Can you work these out from the model? Positions are in its coordinate system, mm. A direction names the side the tool comes from. Give positions to 0.01 mm unless a question says otherwise; leave off trailing zeros. Order: outer loops, then holes, each group sorted by start corner. A loop starts at its lowest first (then second) coordinate and runs counter-clockwise, first axis right, second up.
Item 1: I want a section at D-D, the plane y = -1. Write out the boundary of the cut face in (x, z), then the cut area to 3 significant figures.
Item 2: If we mould it in two halves opening along Y, with no side actions, what happens to faces 5 (the flat face through (-37, 0, 32.5)), 6 (the flat face through (-37, 10, 64.2)), 7 (the flat face through (-37, -15.45, 54)), 8 (the cylindrical face through (-37.48, 10.45, 37.38))? For each: +Y half, -Y half, draft (parallel to the pull), parting line (faces both ways), or undercut.
Item 3: Which directions (+Z, -Z, +X, -X, +Y, -Y) give clear straight access to the entire face, cutting with the end or side of a thin tool? Please do faces 1 (the flat face through (-35, 5, 45)), 2 (the flat face through (-32, 7.5, 66)), 3 (the flat face through (-57.5, 0, 51)), 4 (the flat face through (-56, 0, 52.1)).
Item 4: I want a section at A-A, the plane z = 54.5. Write out the boundary of the cut face in (x, y).
Item 5: I want a section at B-B, the plane x = -21. Write out the boundary of the cut face in (y, z).
Item 6: I'm going to push flat-ended pins straight in: pin 1 Ø4 at (y, z) = (-1, 40) entering from +X; pin 2 Ø2 at (y, z) = (0.5, 48.5) entering from +X; pin 3 Ø1.5 at (x, y) = (-44.5, -0.5) entering from +Z. Where does each tip first touch, or does it pass through?
Item 7: If I drill on line 1 along Y through (x, z) = (-48, 50.5); line 2 along Z through (x, y) = (-35, -0.5); line 3 along Z through (x, y) = (-50.5, -9.5), over which ranges is the centre line in solid material (lowest first)?
Item 8: I want a section at C-C, the plane z = 45.5. Write out the boundary of the cut face in (x, y).
```python
from build123d import *

# Parameters (mm, degrees)
SKETCH1_W               = 115
SKETCH1_H               = 90
BOSS_EXTRUDE1_DEPTH     = 2.5
SKETCH2_W               = 27.2
SKETCH2_H               = 30.9
SKETCH2_W_2             = 19.2
SKETCH2_H_2             = 22.9
BOSS_EXTRUDE2_DEPTH     = 40.6
SKETCH3_W               = 19.2
SKETCH3_H               = 22.9
BOSS_EXTRUDE3_DEPTH     = 4
CUT_EXTRUDE1_REACH      = 136.592
SKETCH4_W               = 5
SKETCH4_H               = 8
FILLET1_R               = 25
SKETCH5_W               = 38.2
SKETCH5_H               = 8
CUT_EXTRUDE2_DEPTH      = 39.6
CUT_EXTRUDE3_REACH      = 92.993
SKETCH6_W               = 20
SKETCH6_H               = 9.5
CUT_EXTRUDE4_REACH      = 129.903
CUT_EXTRUDE5_DEPTH      = 135.591762378
CUT_EXTRUDE5_DEPTH_BACK = 135.591762378
SKETCH9_W               = 100.7
SKETCH9_H               = 30.9
CUT_EXTRUDE6_REACH      = 92.993


# Read off the part's stored shape, not the designer's step: Mirror1
with BuildPart() as part:
    # Sketch1 → Boss-Extrude1 (new, symmetric)
    with BuildSketch(Plane(origin=(0, 0, 0), x_dir=(1, 0, 0), z_dir=(0, 1, 0))):
        Rectangle(SKETCH1_W, SKETCH1_H)
    extrude(amount=BOSS_EXTRUDE1_DEPTH, both=True)

    # Sketch2 → Boss-Extrude2 (add)
    with BuildSketch(Plane.ZY.offset(57.5)):
        with Locations((54.6, 0)):
            Rectangle(SKETCH2_W, SKETCH2_H)
        with Locations((54.6, 0)):
            Rectangle(SKETCH2_W_2, SKETCH2_H_2, mode=Mode.SUBTRACT)
    extrude(amount=-BOSS_EXTRUDE2_DEPTH)

    # Sketch3 → Boss-Extrude3 (add)
    with BuildSketch(Plane.ZY.offset(57.5)):
        with Locations((54.6, 0)):
            Rectangle(SKETCH3_W, SKETCH3_H)
    extrude(amount=-BOSS_EXTRUDE3_DEPTH)

    # Sketch4 → Cut-Extrude1 (cut, up to next)
    with BuildSketch(Plane.ZY.offset(57.5), mode=Mode.PRIVATE) as cut_extrude1_sk1:
        with Locations((54.6, 0)):
            Rectangle(SKETCH4_W, SKETCH4_H)
    cut_extrude1_tool1 = extrude(cut_extrude1_sk1.sketch, amount=-CUT_EXTRUDE1_REACH, mode=Mode.PRIVATE) & part.part
    add(cut_extrude1_tool1.solids().sort_by_distance((-57.5, 0, 54.6))[0], mode=Mode.SUBTRACT)

    # Fillet1
    # the kernel refuses this fillet: 25 mm, written as the material it adds along each edge
    with BuildSketch(Plane(origin=(-57.5, -2.5, 41), x_dir=(0, 0, -1), z_dir=(1, 0, 0))) as fillet1_piece_1:
        with BuildLine():
            CenterArc((21.904280404, -25), FILLET1_R, 90, 61.183893167)
            Line((0, -12.95), (-0.438085608, -12.709))
            ThreePointArc((-0.438085608, -12.709), (-0.5, -6.475), (-0.5, 0))
            Line((-0.5, 0), (0, 0.5))
            Line((0, 0.5), (21.904280404, 0.5))
            Line((21.904280404, 0.5), (21.904280404, 0))
        make_face()
    extrude(amount=40.6)
    with BuildSketch(Plane(origin=(-57.5, 2.5, 41), x_dir=(0, 0, -1), z_dir=(1, 0, 0))) as fillet1_piece_2:
        with BuildLine():
            CenterArc((21.904280404, 25), FILLET1_R, 208.816106833, 61.183893167)
            Line((0, 12.95), (-0.438085608, 12.709))
            ThreePointArc((-0.438085608, 12.709), (-0.5, 6.475), (-0.5, 0))
            Line((-0.5, 0), (0, -0.5))
            Line((0, -0.5), (21.904280404, -0.5))
            Line((21.904280404, -0.5), (21.904280404, 0))
        make_face()
    extrude(amount=40.6)

    # Sketch5 → Cut-Extrude2 (cut)
    with BuildSketch(Plane(origin=(-8.9, 0, 0), x_dir=(0, 0, -1), z_dir=(1, 0, 0))):
        with Locations((-54.6, 0)):
            Rectangle(SKETCH5_W, SKETCH5_H)
    extrude(amount=-CUT_EXTRUDE2_DEPTH, mode=Mode.SUBTRACT)

    # Sketch6 → Cut-Extrude3 (cut, up to next)
    with BuildSketch(Plane(origin=(0, 2.5, 0), x_dir=(1, 0, 0), z_dir=(0, 1, 0)), mode=Mode.PRIVATE) as cut_extrude3_sk1:
        with Locations((1.1, -40.25)):
            Rectangle(SKETCH6_W, SKETCH6_H)
    cut_extrude3_tool1 = extrude(cut_extrude3_sk1.sketch, amount=-CUT_EXTRUDE3_REACH, mode=Mode.PRIVATE) & part.part
    add(cut_extrude3_tool1.solids().sort_by_distance((1.1, 2.5, 40.25))[0], mode=Mode.SUBTRACT)

    # Sketch8 → Cut-Extrude4 (cut, up to next)
    with BuildSketch(Plane.XY.offset(68.2), mode=Mode.PRIVATE) as cut_extrude4_sk1:
        with BuildLine():
            Line((-46, 7.5), (-16, 7.5))
            ThreePointArc((-16, 7.5), (-8.5, 0), (-16, -7.5))
            Line((-16, -7.5), (-46, -7.5))
            ThreePointArc((-46, -7.5), (-53.5, 0), (-46, 7.5))
        make_face()
    cut_extrude4_tool1 = extrude(cut_extrude4_sk1.sketch, amount=-CUT_EXTRUDE4_REACH, mode=Mode.PRIVATE) & part.part
    add(cut_extrude4_tool1.solids().sort_by_distance((-31, 0, 68.2))[0], mode=Mode.SUBTRACT)

    # Mirror1
    split(bisect_by=Plane.XY, keep=Keep.TOP)

    # Mirror1 2: part across plane


with BuildPart() as part_1:
    add(part.part)
    add(part.part.mirror(Plane.XY))

    # Sketch9 → Cut-Extrude5 (cut, two sides: drawn at the far end of the back side and taken through both)
    with BuildSketch(Plane(origin=(57.5, 0, 0), x_dir=(0, 0, -1), z_dir=(1, 0, 0)).offset(-CUT_EXTRUDE5_DEPTH_BACK)):
        with Locations((17.85, 0)):
            Rectangle(SKETCH9_W, SKETCH9_H)
    extrude(amount=CUT_EXTRUDE5_DEPTH + CUT_EXTRUDE5_DEPTH_BACK, mode=Mode.SUBTRACT)

    # Sketch10 → Cut-Extrude6 (cut, up to next)
    with BuildSketch(Plane(origin=(0, 2.5, 0), x_dir=(1, 0, 0), z_dir=(0, 1, 0)), mode=Mode.PRIVATE) as cut_extrude6_sk1:
        Polygon((57.5, -32.5), (-16.9, -32.5), (-16.9, -35.5), (11.1, -35.5), (11.1, -45), (57.5, -45), align=None)
    cut_extrude6_tool1 = extrude(cut_extrude6_sk1.sketch, amount=-CUT_EXTRUDE6_REACH, mode=Mode.PRIVATE) & part_1.part
    add(cut_extrude6_tool1.solids().sort_by_distance((29.593976, 2.5, 38.149096))[0], mode=Mode.SUBTRACT)


solid = part_1.part
```
Results list:
1. outline: (-57.5, 32.5) - (-16.9, 32.5) - (-16.9, 35.5) - (-48.5, 35.5) - (-48.5, 45) - (-53.5, 45) - (-53.5, 52.1) - (-57.5, 52.1) - close; (-57.5, 57.1) - (-53.5, 57.1) - (-53.5, 64.2) - (-53.43, 64.2) - (-53.43, 68.2) - (-57.5, 68.2) - close
1. area: 280 mm2
2. face 5: draft
2. face 6: undercut
2. face 7: -Y half
2. face 8: +Y half
3. face 1: +X
3. face 2: +Z, +X
3. face 3: +Z, -Z, -X, +Y, -Y
3. face 4: +X, -X
4. outline: (-57.5, -15.45) - (-16.9, -15.45) - (-16.9, -11.45) - (-53.5, -11.45) - (-53.5, -4) - (-57.5, -4) - close; (-57.5, 4) - (-53.5, 4) - (-53.5, 11.45) - (-16.9, 11.45) - (-16.9, 15.45) - (-57.5, 15.45) - close
5. outline: (-15.45, 41) arc R25 cw to (-6.4, 32.5) - (6.4, 32.5) arc R25 cw to (15.45, 41) - (15.45, 68.2) - (7.5, 68.2) - (7.5, 64.2) - (11.45, 64.2) - (11.45, 45) - (4, 45) - (4, 35.5) - (-4, 35.5) - (-4, 45) - (-11.45, 45) - (-11.45, 64.2) - (-7.5, 64.2) - (-7.5, 68.2) - (-15.45, 68.2) - close
6. pin 1: stops at x = -48.5
6. pin 2: stops at x = -53.5
6. pin 3: stops at z = 35.5
7. line 1: y = -15.45 to -11.45, 11.45 to 15.45
7. line 2: z = 32.5 to 35.5
7. line 3: z = 36.45 to 45, 64.2 to 68.2
8. outline: (-57.5, -15.45) - (-16.9, -15.45) - (-16.9, -11.45) - (-53.5, -11.45) - (-53.5, 11.45) - (-16.9, 11.45) - (-16.9, 15.45) - (-57.5, 15.45) - close
